Input: part model. Units: mm. Frame: model coordinates. Face numbers are marked on the shaded views. Give positions to 0.01 mm unless a question says otherwise; leave off trailing zeros. Loops run counter-clockwise (first coordinate to the right, second up) from the corner with the lowest first, then second, coordinate; pieces in that order, holes last. Notation, with made-up numbers: (45.25, 21.5) -> (50.25, 21.5) arc R26 ccw to (50.25, 35.5) -> close; hole circle Ø8 at (61.25, -32.5). An arc over 180 degrees is marked (long way). Answer in a Markdown table with one row per item. Add a question column.
```python
from build123d import *

# Parameters (mm, degrees)
BOSS_EXTRUDE2_DEPTH = 19.05
BOSS_EXTRUDE3_DEPTH = 6.35
BOSS_EXTRUDE4_DEPTH = 6.35
SKETCH5_R           = 3.175
CUT_EXTRUDE1_DEPTH  = 653.553447442
SKETCH6_R           = 3.175
CUT_EXTRUDE2_DEPTH  = 653.553447442
BOSS_EXTRUDE7_DEPTH = 7.874
SKETCH12_R          = 3.175
CUT_EXTRUDE4_DEPTH  = 675.468016292
BOSS_EXTRUDE8_DEPTH = 23.1648
CUT_EXTRUDE6_DEPTH  = 429.875020033


with BuildPart() as part:
    # Sketch1 → Boss-Extrude2 (new body)
    with BuildSketch(Plane.XY):
        with BuildLine():
            Line((642.224572561, 111.046838573), (634.252545404, 110.925124722))
            ThreePointArc((634.252545404, 110.925124722), (637.340775548, 101.689054702), (630.810820972, 94.46397006))
            Line((630.810820972, 94.46397006), (628.034186285, 94.421577467))
            add(Edge.make_bspline(
                [(623.884527878, 94.077084958), (624.201469176, 94.081923896), (624.52651862, 94.107859076), (625.194071811, 94.176161637), (625.538291649, 94.218971248), (626.23780183, 94.300697743), (626.591177817, 94.339281954), (627.30622807, 94.396985819), (627.667912536, 94.41598534), (628.034186285, 94.421577467)],
                knots=[0, 0, 0, 0, 0.25, 0.25, 0.5, 0.5, 0.75, 0.75, 1, 1, 1, 1], degree=3))
            Line((623.884527878, 94.077084958), (614.502973196, 93.933850981))
            Line((614.502973196, 93.933850981), (614.557258512, 90.378265361))
            Line((614.557258512, 90.378265361), (642.533611114, 90.805397577))
            Line((642.533611114, 90.805397577), (642.224572561, 111.046838573))
        make_face()
    extrude(amount=-BOSS_EXTRUDE2_DEPTH)

    # Sketch2 → Boss-Extrude3 (add)
    with BuildSketch(Plane.XY):
        Polygon((614.557258512, 90.378265361), (614.248219959, 110.619706357), (642.224572561, 111.046838573), (642.533611114, 90.805397577), align=None)
    extrude(amount=BOSS_EXTRUDE3_DEPTH)

    # Sketch4 → Boss-Extrude4 (add)
    with BuildSketch(Plane(origin=(0, 0, -19.05), x_dir=(-1, 0, 0), z_dir=(0, 0, -1))):
        Polygon((-614.557258512, 90.378265361), (-614.248219959, 110.619706357), (-642.224572561, 111.046838573), (-642.533611114, 90.805397577), align=None)
    extrude(amount=BOSS_EXTRUDE4_DEPTH)

    # Sketch5 → Cut-Extrude1 (cut, through all)
    with BuildSketch(Plane(origin=(0, 0, 0), x_dir=(-1, 0, 0), z_dir=(0, 0, -1))):
        with Locations((-627.893070479, 103.664395923)):
            Circle(SKETCH5_R)
    extrude(amount=-CUT_EXTRUDE1_DEPTH, mode=Mode.SUBTRACT)

    # Sketch6 → Cut-Extrude2 (cut, through all)
    with BuildSketch(Plane.XY.offset(-19.05)):
        with Locations(Location((627.893070479, 103.664395923, 0), (0, 0, 180))):
            Circle(SKETCH6_R)
    extrude(amount=-CUT_EXTRUDE2_DEPTH, mode=Mode.SUBTRACT)

    # Sketch11 → Boss-Extrude7 (add)
    with BuildSketch(Plane(origin=(-1.236319125, 80.976565327, 0), x_dir=(0.9998834703189056, 0.015265837121568253, 0), z_dir=(0.015265837121568255, -0.9998834703189057, 0))):
        Polygon((615.865344229, 6.35), (600.772109003, 28.658661472), (619.965955333, 41.644525188), (643.844957287, 6.35), (672.023174673, -35.299010508), (652.829328343, -48.284874224), align=None)
    extrude(amount=BOSS_EXTRUDE7_DEPTH)

    # Sketch12 → Cut-Extrude4 (cut, through all)
    with BuildSketch(Plane(origin=(-1.236319125, 80.976565327, 0), x_dir=(0.9998834703189056, 0.015265837121568083, 0), z_dir=(-0.015265837121568085, 0.9998834703189057, 0))):
        with Locations(Location((618.191262939, -22.963551046, 0), (0, 0, 180))):
            Circle(SKETCH12_R)
        with Locations(Location((654.022628802, 29.997248883, 0), (0, 0, 180))):
            Circle(SKETCH12_R)
    extrude(amount=-CUT_EXTRUDE4_DEPTH, mode=Mode.SUBTRACT)

    # Sketch13 → Boss-Extrude8 (add)
    with BuildSketch(Plane(origin=(444.569112267, 6.787510604, 300.814470562), x_dir=(0.5602970950459771, 0.008554401034284214, -0.8282475399939222), z_dir=(0.8281510245722196, 0.012643892041886809, 0.5603623938970352))):
        Polygon((312.913631323, 73.066855862), (405.705293775, 70.658703567), (405.812833532, 73.1120026), (312.913631323, 73.1120026), align=None)
    extrude(amount=-BOSS_EXTRUDE8_DEPTH)

    # Sketch14 → Cut-Extrude6 (cut, through all)
    with BuildSketch(Plane(origin=(444.569112267, 6.787510604, 300.814470562), x_dir=(0.5602970950459771, 0.008554401034284214, -0.8282475399939222), z_dir=(0.8281510245722196, 0.012643892041886809, 0.5603623938970352))):
        Polygon((312.913631323, 73.066855862), (312.913631323, 77.045511862), (405.812833532, 74.637359567), (405.705293775, 70.658703567), align=None)
    extrude(amount=-CUT_EXTRUDE6_DEPTH, mode=Mode.SUBTRACT)


with BuildPart() as body_2:
    # of the pieces the cut leaves, the one that is kept (cut_extrude6_keep)
    add(part.part.solids().sort_by_distance((634.252545404, 110.925124722, 0))[0])


solid = body_2.part
```
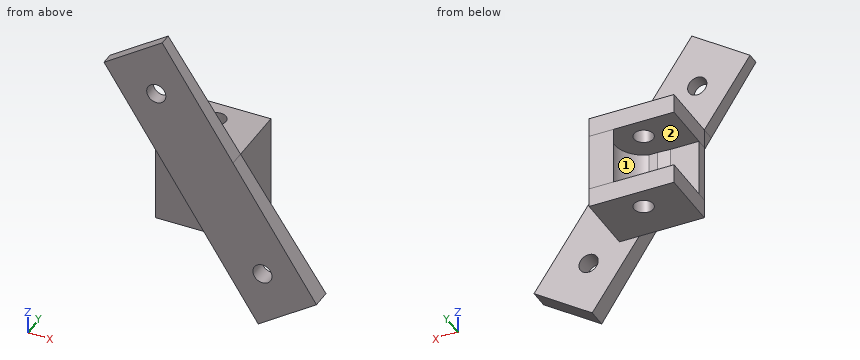
1) Section C-C on x = 641. Output: boundary loops of the cut face in (y, z), and give its area (3 significant figures).
2) Section D-D on y = 97.25. Output: boundary loops of the cut face in (x, z).
3) Pin query (flat end, axial travel): pin 1 (6 mm diameter, centred on y = 94, z = -10.5, fed in from -X); pin 2 (6 mm diameter, centred on x = 631.5, y = 97.5, fed in from -Z); pin 3 (4 mm diameter, centred on x = 620, z = -15.5, fed in from +Y); pin 4 (5 mm diameter, centred on x = 627.89, y = 103.66, fed in from -Z). Return the tip coordinate at first contact, or that it passes through.
4) Material intervals for line 1 along Z through (x, y) = (624, 98.25); line 2 along Y through (x, z) = (615, -22); line 3 along X through (y, z) = (91.25, 0.5), sorted ascending.
5) Section A-A on z = -28.5. Output: boundary loops of the cut face in (x, y), and give its area (3 significant figures).
6) Section B-B on y = 105.5. Output: boundary loops of the cut face in (x, z), and give its area (3 significant figures).
7) Pull-direction query (X, two-part tool) for the marked faces 1 and 2; classes: +X half, -X half, draft (parallel to the pull), parting line (faces both ways), or undercut.
Working result:
| question | item | result |
|---|---|---|
| 1 | outline | (84.92, -32.61) -> (90.78, -32.74) -> (90.78, -25.4) -> (111.03, -25.4) -> (111.03, 6.35) -> (90.78, 6.35) -> (90.78, 8.62) -> (85.81, 8.73) -> close |
| 1 | area | 867 mm2 |
| 2 | outline | (614.45, -25.4) -> (642.44, -25.4) -> (642.44, 6.35) -> (614.45, 6.35) -> (614.45, 0) -> (635.11, 0) -> (635.11, -19.05) -> (614.45, -19.05) -> close |
| 3 | pin 1 | stops at x = 614.5 |
| 3 | pin 2 | stops at z = -25.4 |
| 3 | pin 3 | stops at y = 94.05 |
| 3 | pin 4 | passes through |
| 4 | line 1 | z = -25.4 to -19.05, 0 to 6.35 |
| 4 | line 2 | y = 90.39 to 110.63 |
| 4 | line 3 | x = 614.54 to 642.53 |
| 5 | outline | (638.13, 90.74) -> (638.22, 85.01) -> (650, 85.02) -> (649.91, 90.92) -> close; (655.51, 91) -> (655.6, 85.02) -> (666.2, 85.03) -> (666.11, 91.17) -> close |
| 5 | area | 133 mm2 |
| 6 | outline | (614.33, -25.4) -> (625.3, -25.4) -> (625.3, -19.05) -> (614.33, -19.05) -> close; (614.33, 0) -> (625.3, 0) -> (625.3, 6.35) -> (614.33, 6.35) -> close; (630.48, -25.4) -> (642.31, -25.4) -> (642.31, 6.35) -> (630.48, 6.35) -> (630.48, 0) -> (637.37, 0) -> (637.37, -19.05) -> (630.48, -19.05) -> close |
| 6 | area | 384 mm2 |
| 7 | face 1 | -X half |
| 7 | face 2 | draft |
